```python
from build123d import *

# Parameters (mm, degrees)
F1_DEPTH = 10
F2_R     = 5.08
F4_DEPTH = 60
F5_R     = 5.08
F7_DEPTH = 5.08
F8_R     = 5.08


# Not quite as in the source:
# - a feature names something its author has since deleted; it is built from what else it names


with BuildPart() as f1:
    # F0 (on Top) → F1 (new body)
    with BuildSketch(Plane.XY):
        Polygon((63.5, 38.1), (63.5, 63.5), (38.1, 63.5), (50.8, 50.8), align=None)
        Polygon((50.8, 50.8), (38.1, 63.5), (-50.8, 63.5), (-50.8, 32.8394877579), (32.8394877579, -50.8), (63.5, -50.8), (63.5, 38.1), align=None)
        Polygon((-50.8, 32.8394877579), (-50.8, 63.5), (-81.4605122421, 63.5), align=None)
        Polygon((63.5, -81.4605122421), (63.5, -50.8), (32.8394877579, -50.8), align=None)
    extrude(amount=F1_DEPTH)

    # F2
    f2_edges = [f1.edges().sort_by_distance(p)[0] for p in [
        (63.5, -81.460512, 5),
        (-81.460512, 63.5, 5),
        (63.5, 63.5, 5),
    ]]
    fillet(f2_edges, radius=F2_R)

    # F0 (on Top) + F3 (on face) → F4 (join)
    with BuildSketch(Plane.XY):
        Polygon((63.5, -81.4605122421), (63.5, -50.8), (32.8394877579, -50.8), align=None)
        Polygon((63.5, 38.1), (63.5, 63.5), (38.1, 63.5), (50.8, 50.8), align=None)
    with BuildSketch(Plane.XY):
        Polygon((-50.8, 63.5), (-81.4605122421, 63.5), (-50.8, 32.8394877579), align=None)
    extrude(amount=-F4_DEPTH)

    # F5
    f5_edges = [f1.edges().sort_by_distance(p)[0] for p in [
        (-81.460512, 63.5, -30),
        (63.5, -81.460512, -30),
        (63.5, 63.5, -30),
        (32.839488, -50.8, -30),
        (-50.8, 32.839488, -30),
        (-50.8, 63.5, -30),
        (38.1, 63.5, -30),
        (63.5, 38.1, -30),
        (63.5, -50.8, -30),
    ]]
    fillet(f5_edges, radius=F5_R)

    # F6 (on face) → F7 (cut)
    with BuildSketch(Plane.XY.offset(10)):
        Polygon((50.8, 50.8), (-50.8, 50.8), (50.8, -50.8), align=None)
    extrude(amount=-F7_DEPTH, mode=Mode.SUBTRACT)

    # F8
    f8_edges = [f1.edges().sort_by_distance(p)[0] for p in [
        (50.8, 50.8, 7.46),
        (-50.8, 50.8, 7.46),
        (50.8, -50.8, 7.46),
    ]]
    fillet(f8_edges, radius=F8_R)


solid = f1.part
```
Part model, mm, in its own coordinate system. A direction names the side the tool comes from. Coordinates: 2 decimals unless noted, no trailing zeros. Order: outer loops, then holes, each group sorted by start corner. A loop starts at its lowest first (then second) coordinate and runs counter-clockwise, first axis right, second up. Notation, with made-up numbers: (84, -13.75) - (141, -13.75) arc R33 ccw to (141, 23.25) - close; hole circle Ø8 at (-34.5, -3.75). An arc over 180 degrees is marked (long way). Return JSON: item names as keys, results as strings. Group by question number.
Item 1: Pull direction Y, two halves, no side cores. Call faces 1 (the face through (-60, 55, -60)), 2 (the face through (50.7, 50.9, -29.6)), 3 (the face through (62.051, 61.972, -30.42)): pulls with the +Y half, pulls with the -Y half, needs draft (parallel to the pull), parting line crosses it, or undercut.
Item 2: Cut at B-B (y = -6). List the corners of the cut face in (x, z).
Item 3: Cut at C-C (x = 16). List the corners of the cut face in (y, z).
Item 4: Drill centre lines: probe 1 along Y at (x, z) = (55.5, -18); probe 2 along Z at (x, y) = (-27.5, 47); probe 3 along Z at (x, y) = (-32.5, 54). Where is each one in solid material? Low to high. Write a range as from..to.
Item 5: Cut at D-D (y = -64). List the corners of the cut face in (x, z), plus the area to 3 significant figures.
Item 6: Which spindle directions (+Z, -Z, +X, -X, +Y, -Y) get a long thin tool onto all of the face, cutting with end or side? Do faces 4 (the face through (-52.249, 61.972, -30.42)), 5 (the face through (40.38, -54.01, -30.42)), 6 (the face through (-54.01, 40.38, -30.42)). Say none if no direction does.
Item 7: Cut at A-A (z = -42). List the corners of the cut face in (x, y).
Item 8: Pin check, flat tips, straight feed: pin 1 (5.5 mm diameter, centred on y = 22, z = 7, fed in from -X); pin 2 (1.5 mm diameter, centred on x = -11, z = 7, fed in from -Y); pin 3 (1 mm diameter, centred on x = 36.5, y = 27, fed in from -Z). Stop position of each tip, or through.
Check values:
{
 "1": {"face 1": "needs draft", "face 2": "undercut", "face 3": "pulls with the +Y half"},
 "2": {"outline": "(-11.96, 0) - (63.5, 0) - (63.5, 10) - (50.8, 10) - (50.8, 4.92) - (6, 4.92) - (6, 10) - (-11.96, 10) - close"},
 "3": {"outline": "(-33.96, 0) - (63.5, 0) - (63.5, 10) - (50.8, 10) - (50.8, 4.92) - (-16, 4.92) - (-16, 10) - (-33.96, 10) - close"},
 "4": {"probe 1": "y = -73.35..-50.8, 46.21..63.5", "probe 2": "z = 0..4.92", "probe 3": "z = 0..10"},
 "5": {"outline": "(46.04, -60) - (63.5, -60) - (63.5, 10) - (46.04, 10) - close", "area": "1,220 mm2"},
 "6": {"face 4": "-Z, +Y", "face 5": "-Z, -X", "face 6": "-Z, -Y"},
 "7": {"outline": "(-72.79, 54.83) - (-59.47, 41.51) arc R5.08 ccw to (-50.8, 45.1) - (-50.8, 58.42) arc R5.08 ccw to (-55.88, 63.5) - (-69.2, 63.5) arc R5.08 ccw to start; (41.51, -59.47) - (54.83, -72.79) arc R5.08 ccw to (63.5, -69.2) - (63.5, -55.88) arc R5.08 ccw to (58.42, -50.8) - (45.1, -50.8) arc R5.08 ccw to start; (46.77, 54.83) - (54.83, 46.77) arc R5.08 ccw to (63.5, 50.36) - (63.5, 58.42) arc R5.08 ccw to (58.42, 63.5) - (50.36, 63.5) arc R5.08 ccw to start"},
 "8": {"pin 1": "stops at x = -42.71", "pin 2": "stops at y = -7.71", "pin 3": "stops at z = 0"}
}
